```python
from build123d import *

# Parameters (mm, degrees)
SKETCH1_W           = 42
SKETCH1_H           = 42
BOSS_EXTRUDE1_DEPTH = 21
CHAMFER1_SIZE       = 7
FILLET1_R           = 2


with BuildPart() as part:
    # Sketch1 → Boss-Extrude1 (new body)
    with BuildSketch(Plane(origin=(0, 0, 0), x_dir=(1, 0, 0), z_dir=(0, 1, 0))):
        Rectangle(SKETCH1_W, SKETCH1_H)
    extrude(amount=BOSS_EXTRUDE1_DEPTH)

    # Chamfer1
    chamfer1_edges = [part.edges().sort_by_distance(p)[0] for p in [
        (-21, 10.5, -21),
        (21, 10.5, -21),
        (21, 10.5, 21),
        (-21, 10.5, 21),
    ]]
    chamfer(chamfer1_edges, length=CHAMFER1_SIZE)

    # Fillet1
    fillet1_edges = [part.edges().sort_by_distance(p)[0] for p in [
        (-21, 10.5, 14),
        (-21, 10.5, -14),
        (-14, 10.5, -21),
    ]]
    fillet(fillet1_edges, radius=FILLET1_R)


solid = part.part
```
Could you check a few things on this model? Use its own coordinates, in mm. Round coordinates to 2 decimals unless told otherwise and drop trailing zeros. Loops run counter-clockwise (first coordinate to the right, second up) from the corner with the lowest first, then second, coordinate; pieces in that order, holes last. Notation, with made-up numbers: M 72,-19 L 79,-19 A29 ccw 79,16 Z; hole C -40,65 d5. An arc over 180 degrees is marked long. Write item = value, one per line.
1. I want a section at A-A, the plane y = 6.5. Write out the boundary of the cut face in (x, z).
Results below:
outline = M -21,-13.17 A2 ccw -20.41,-14.59 L -14.59,-20.41 A2 ccw -13.17,-21 L 14,-21 L 21,-14 L 21,14 L 14,21 L -14,21 L -20.41,14.59 A2 ccw -21,13.17 Z
2. I need wall thicknesses on probe 1 along X at (y, z) = (3.5, 18); probe 2 along Z at (x, y) = (-15, 6.25); probe 3 along X at (y, z) = (10.5, 15.5). Which ranges of each line are inside material? Lowest first, please.
Results below:
probe_1 = -17 to 17
probe_2 = -20 to 20
probe_3 = -19.5 to 19.5
3. I want a section at B-B, the plane x = 15. Write out the boundary of the cut face in (y, z), and give its area (3 significant figures).
Results below:
outline = M 0,-20 L 21,-20 L 21,20 L 0,20 Z
area = 840 mm²
4. I want a section at C-C, the plane z = 18.5. Write out the boundary of the cut face in (x, y).
Results below:
outline = M -16.5,0 L 16.5,0 L 16.5,21 L -16.5,21 Z
